Geometry check sheet. Reference: the model listing, model coordinates, mm. A direction names the side the tool comes from. Coordinates: 2 decimals unless noted, no trailing zeros. Write each loop counter-clockwise with the first axis right and the second up, starting at its lowest first coordinate (ties: lowest second). Pieces come first, ordered by that corner, then holes. Notation, with made-up numbers: (-4, 37) -> (7, 37) arc R18 ccw to (7, 44) -> close; hole circle Ø2 at (81.5, 5.25). An arc over 180 degrees is marked (long way). Answer in a Markdown table with one row per item. Add a question column.
1. Set-up check for faces 1 (the cylindrical face through (22.5, 21.5, -10)), 2 (the flat face through (0, -18, 14.5)), 3 (the cylindrical face through (22.507, -12.594, -15.281)): record each of +Z, -Z, +X, -X, +Y, -Y from which the full face is reachable in a straight line by a thin tool's end or side.
2. Cross-section at A-A on y = -4.5. Record the cut outline in (x, z).
3. Cross-section at D-D on y = 2. Record the cut outline in (x, z), and give its area (3 significant figures).
4. Mould release check, pull along Z, two halves, no side actions. Record for faces 4 (the flat face through (2, -17, 0)), 5 (the flat face through (20.6, 1, 8)), 6 (the cylindrical face through (14.23, -16.78, -1.97)): pulls with the +Z half, pulls with the -Z half, needs draft (parallel to the pull), parting line crosses it, or undercut.
5. Cross-section at C-C on y = 10. Record the cut outline in (x, z).
6. Cross-section at B-B on x = 0. Record the cut outline in (y, z), and give its area (4 significant figures).
7. Scan lines: L1, parallel to Z at x = -18, y = -17; L2, parallel to X at y = -10, z = 7; L3, parallel to X at y = -16, z = -9.5. Record each from-to range of solid material in increasing order. Write a range as from..to.
8. Depth check by flat-ended pin: P1, Ø0.8, axis at x = 22.5, y = 5, coming from the -Z side; P2, Ø2.5, axis at x = 22, z = 5.5, coming from the +Y side; P3, Ø0.5, axis at x = 22.5, z = -48, coming from the +Y side. Enter the tip coordinate at first touch or a pass-through.
```python
from build123d import *

# Parameters (mm, degrees)
F0_W         = 44
F0_H         = 42
F1_DEPTH     = 1
F3_DEPTH     = 13.5
F4_W         = 41.2
F4_H         = 40.1
F5_DEPTH     = 1
F7_DEPTH     = 25
F9_DEPTH     = 1
F11_DEPTH    = 25
F12_W        = 42
F12_H        = 15.5
F12_W_2      = 1
F12_H_2      = 9
F13_DEPTH    = 1
F14_DEPTH    = 25
F15_R        = 8
F16_T1_DEPTH = 1
F16_T3_DEPTH = 11
F16_T5_DEPTH = 11
F16_T7_DEPTH = 11
F16_T9_DEPTH = 11
F8_R         = 1.25
F17_DEPTH    = 5
F18_R        = 1


# Not quite as in the source:
# - a fillet or chamfer that OpenCascade refuses, or shapes differently, is made with other operations: its cross-section is extruded or revolved along the edge and cut away or added
# - a feature names something its author has since deleted; it is built from what else it names


with BuildPart() as f1:
    # F0 (on Top) → F1 (new body)
    with BuildSketch(Plane.XY):
        Rectangle(F0_W, F0_H)
    extrude(amount=F1_DEPTH)

    # F2 (on face) → F3 (join)
    with BuildSketch(Plane.XY.offset(1)):
        Polygon((-20.6, -19.1), (-20.6, 21), (-22, 21), (-22, -21), (22, -21), (22, 21), (20.6, 21), (20.6, -19.1), align=None)
    extrude(amount=F3_DEPTH)

    # F4 (on face) → F5 (join)
    with BuildSketch(Plane.XY.offset(14.5)):
        with Locations((0, 0.95)):
            Rectangle(F4_W, F4_H)
        Polygon((-22, 21), (-22, -21), (22, -21), (22, 21), (20.6, 21), (20.6, -19.1), (-20.6, -19.1), (-20.6, 21), align=None)
    extrude(amount=F5_DEPTH)

    # F6 (on face) → F7 (cut, symmetric)
    with BuildSketch(Plane.XY.offset(1)):
        with BuildLine():
            ThreePointArc((-20.6, 4.0000000362), (-1.81e-08, -16.6), (20.6, 4))
            ThreePointArc((20.6, 4), (18.2212690578, 13.6096490011), (11.6344316578, 21))
            Line((11.6344316578, 21), (-11.6344316578, 21))
            ThreePointArc((-11.6344316578, 21), (-18.2212690493, 13.6096490171), (-20.6, 4.0000000362))
        make_face()
        with BuildLine():
            Line((-20.6, 21), (-20.6, 4.0000000362))
            ThreePointArc((-20.6, 4.0000000362), (-18.2212690493, 13.6096490171), (-11.6344316578, 21))
            Line((-11.6344316578, 21), (-20.6, 21))
        make_face()
        with BuildLine():
            ThreePointArc((11.6344316578, 21), (18.2212690578, 13.6096490011), (20.6, 4))
            Line((20.6, 4), (20.6, 21))
            Line((20.6, 21), (11.6344316578, 21))
        make_face()
    extrude(amount=F7_DEPTH, both=True, mode=Mode.SUBTRACT)

    # F4 (on face) → F9 (join)
    with BuildSketch(Plane.XY.offset(14.5)):
        Polygon((-22, 21), (-22, -21), (22, -21), (22, 21), (20.6, 21), (20.6, -19.1), (-20.6, -19.1), (-20.6, 21), align=None)
    extrude(amount=F9_DEPTH)

    # F10 (on face) → F11 (cut)
    with BuildSketch(Plane.YZ.offset(-20.6)):
        Polygon((21, 0), (21, 15), (21, 15.5), (4, 15.5), (4, 14.5), (4, 1), (4, 0), align=None)
    extrude(amount=-F11_DEPTH, mode=Mode.SUBTRACT)

    # F12 (on face) → F13 (join)
    with BuildSketch(Plane.YZ.offset(22)):
        Polygon((21, 0), (-21, 0), (-21, -13), (-15, -13), (25, -13), (25, 0), align=None)
        with BuildLine():
            Line((23, -7.5), (23, -8.5))
            ThreePointArc((23, -8.5), (21.5, -10), (20, -8.5))
            Line((20, -8.5), (20, -7.5))
            ThreePointArc((20, -7.5), (21.5, -6), (23, -7.5))
        make_face(mode=Mode.SUBTRACT)
        Polygon((-15, -13), (-21, -13), (-21, -55), (-15, -55), (-15, -46), align=None)
        with BuildLine():
            Line((-16.45, -49.5), (-16.45, -50.5))
            ThreePointArc((-16.45, -50.5), (-18, -52.05), (-19.55, -50.5))
            Line((-19.55, -50.5), (-19.55, -49.5))
            ThreePointArc((-19.55, -49.5), (-18, -47.95), (-16.45, -49.5))
        make_face(mode=Mode.SUBTRACT)
        with Locations((0, 7.75)):
            Rectangle(F12_W, F12_H)
        with Locations((-14.5, -50.5)):
            Rectangle(F12_W_2, F12_H_2)
    extrude(amount=F13_DEPTH)

    # F12 (on face) → F14 (cut)
    with BuildSketch(Plane.YZ.offset(22)):
        with BuildLine():
            ThreePointArc((-19.55, -50.5), (-18, -52.05), (-16.45, -50.5))
            Line((-16.45, -50.5), (-16.8157280718, -50.5))
            ThreePointArc((-16.8157280718, -50.5), (-18, -51.05), (-19.1842719282, -50.5))
            Line((-19.1842719282, -50.5), (-19.55, -50.5))
        make_face()
        with BuildLine():
            Line((-16.8157280718, -50.5), (-16.45, -50.5))
            ThreePointArc((-16.45, -50.5), (-16.4708552854, -50.2465903676), (-16.5328599249, -50))
            ThreePointArc((-16.5328599249, -50), (-16.6509275769, -50.2632192327), (-16.8157280718, -50.5))
        make_face()
        with BuildLine():
            ThreePointArc((-16.5328599249, -50), (-16.4708552854, -50.2465903676), (-16.45, -50.5))
            Line((-16.45, -50.5), (-16.45, -49.5))
            ThreePointArc((-16.45, -49.5), (-16.4708552854, -49.7534096324), (-16.5328599249, -50))
        make_face()
        with BuildLine():
            ThreePointArc((-16.5328599249, -50), (-16.4708552854, -49.7534096324), (-16.45, -49.5))
            Line((-16.45, -49.5), (-16.8157280718, -49.5))
            ThreePointArc((-16.8157280718, -49.5), (-16.6509275769, -49.7367807673), (-16.5328599249, -50))
        make_face()
        with BuildLine():
            Line((-16.8157280718, -49.5), (-16.45, -49.5))
            ThreePointArc((-16.45, -49.5), (-18, -47.95), (-19.55, -49.5))
            Line((-19.55, -49.5), (-19.1842719282, -49.5))
            ThreePointArc((-19.1842719282, -49.5), (-18, -48.95), (-16.8157280718, -49.5))
        make_face()
        with BuildLine():
            Line((-19.1842719282, -49.5), (-16.8157280718, -49.5))
            ThreePointArc((-16.8157280718, -49.5), (-18, -48.95), (-19.1842719282, -49.5))
        make_face()
        with BuildLine():
            Line((-19.1842719282, -50.5), (-16.8157280718, -50.5))
            ThreePointArc((-16.8157280718, -50.5), (-16.6509275769, -50.2632192327), (-16.5328599249, -50))
            ThreePointArc((-16.5328599249, -50), (-16.6509275769, -49.7367807673), (-16.8157280718, -49.5))
            Line((-16.8157280718, -49.5), (-19.1842719282, -49.5))
            ThreePointArc((-19.1842719282, -49.5), (-19.3490724231, -49.7367807673), (-19.4671400751, -50))
            ThreePointArc((-19.4671400751, -50), (-19.3490724231, -50.2632192327), (-19.1842719282, -50.5))
        make_face()
        with BuildLine():
            ThreePointArc((-19.1842719282, -50.5), (-18, -51.05), (-16.8157280718, -50.5))
            Line((-16.8157280718, -50.5), (-19.1842719282, -50.5))
        make_face()
        with BuildLine():
            ThreePointArc((-19.4671400751, -50), (-19.5291447146, -50.2465903676), (-19.55, -50.5))
            Line((-19.55, -50.5), (-19.1842719282, -50.5))
            ThreePointArc((-19.1842719282, -50.5), (-19.3490724231, -50.2632192327), (-19.4671400751, -50))
        make_face()
        with BuildLine():
            Line((-19.55, -49.5), (-19.55, -50.5))
            ThreePointArc((-19.55, -50.5), (-19.5291447146, -50.2465903676), (-19.4671400751, -50))
            ThreePointArc((-19.4671400751, -50), (-19.5291447146, -49.7534096324), (-19.55, -49.5))
        make_face()
        with BuildLine():
            Line((-19.1842719282, -49.5), (-19.55, -49.5))
            ThreePointArc((-19.55, -49.5), (-19.5291447146, -49.7534096324), (-19.4671400751, -50))
            ThreePointArc((-19.4671400751, -50), (-19.3490724231, -49.7367807673), (-19.1842719282, -49.5))
        make_face()
        with BuildLine():
            ThreePointArc((20, -8.5), (21.5, -10), (23, -8.5))
            Line((23, -8.5), (22.6180339887, -8.5))
            ThreePointArc((22.6180339887, -8.5), (21.5, -9), (20.3819660113, -8.5))
            Line((20.3819660113, -8.5), (20, -8.5))
        make_face()
        with BuildLine():
            ThreePointArc((20.0857864376, -8), (20.0216021605, -8.2463470319), (20, -8.5))
            Line((20, -8.5), (20.3819660113, -8.5))
            ThreePointArc((20.3819660113, -8.5), (20.209430585, -8.2644805982), (20.0857864376, -8))
        make_face()
        with BuildLine():
            Line((20.3819660113, -7.5), (20, -7.5))
            ThreePointArc((20, -7.5), (20.0216021605, -7.7536529681), (20.0857864376, -8))
            ThreePointArc((20.0857864376, -8), (20.209430585, -7.7355194018), (20.3819660113, -7.5))
        make_face()
        with BuildLine():
            Line((22.6180339887, -7.5), (23, -7.5))
            ThreePointArc((23, -7.5), (21.5, -6), (20, -7.5))
            Line((20, -7.5), (20.3819660113, -7.5))
            ThreePointArc((20.3819660113, -7.5), (21.5, -7), (22.6180339887, -7.5))
        make_face()
        with BuildLine():
            Line((20.3819660113, -7.5), (22.6180339887, -7.5))
            ThreePointArc((22.6180339887, -7.5), (21.5, -7), (20.3819660113, -7.5))
        make_face()
        with BuildLine():
            Line((20.3819660113, -8.5), (22.6180339887, -8.5))
            ThreePointArc((22.6180339887, -8.5), (22.790569415, -8.2644805982), (22.9142135624, -8))
            ThreePointArc((22.9142135624, -8), (22.790569415, -7.7355194018), (22.6180339887, -7.5))
            Line((22.6180339887, -7.5), (20.3819660113, -7.5))
            ThreePointArc((20.3819660113, -7.5), (20.209430585, -7.7355194018), (20.0857864376, -8))
            ThreePointArc((20.0857864376, -8), (20.209430585, -8.2644805982), (20.3819660113, -8.5))
        make_face()
        with BuildLine():
            ThreePointArc((20.3819660113, -8.5), (21.5, -9), (22.6180339887, -8.5))
            Line((22.6180339887, -8.5), (20.3819660113, -8.5))
        make_face()
        with BuildLine():
            ThreePointArc((22.9142135624, -8), (22.9783978395, -8.2463470319), (23, -8.5))
            Line((23, -8.5), (23, -7.5))
            ThreePointArc((23, -7.5), (22.9783978395, -7.7536529681), (22.9142135624, -8))
        make_face()
        with BuildLine():
            ThreePointArc((22.9142135624, -8), (22.9783978395, -7.7536529681), (23, -7.5))
            Line((23, -7.5), (22.6180339887, -7.5))
            ThreePointArc((22.6180339887, -7.5), (22.790569415, -7.7355194018), (22.9142135624, -8))
        make_face()
        with BuildLine():
            Line((22.6180339887, -8.5), (23, -8.5))
            ThreePointArc((23, -8.5), (22.9783978395, -8.2463470319), (22.9142135624, -8))
            ThreePointArc((22.9142135624, -8), (22.790569415, -8.2644805982), (22.6180339887, -8.5))
        make_face()
        with BuildLine():
            Line((20, -7.5), (20, -8.5))
            ThreePointArc((20, -8.5), (20.0216021605, -8.2463470319), (20.0857864376, -8))
            ThreePointArc((20.0857864376, -8), (20.0216021605, -7.7536529681), (20, -7.5))
        make_face()
    extrude(amount=-F14_DEPTH, mode=Mode.SUBTRACT)

    # F15
    f15_edges = [f1.edges().sort_by_distance(p)[0] for p in [
        (22.5, -15, -13),
    ]]
    fillet(f15_edges, radius=F15_R)

    # F16: fillet of radius 2 on 5 edges, made by hand

    # F16_s2 → F16_t1 (join)
    with BuildSketch(Plane.YZ.offset(22)):
        with BuildLine():
            ThreePointArc((-15, -44.2679491924), (-14.7320508076, -45.2679491924), (-14, -46))
            Line((-14, -46), (-15, -46))
            Line((-15, -46), (-15, -44.2679491924))
        make_face()
    extrude(amount=F16_T1_DEPTH)

    # F16_s4 → F16_t3 (cut)
    with BuildSketch(Plane.YZ.offset(17)):
        with BuildLine():
            ThreePointArc((23, -13), (24.4142135624, -12.4142135624), (25, -11))
            Line((25, -11), (25, -13))
            Line((25, -13), (23, -13))
        make_face()
    extrude(amount=F16_T3_DEPTH, mode=Mode.SUBTRACT)

    # F16_s6 → F16_t5 (cut)
    with BuildSketch(Plane.YZ.offset(17)):
        with BuildLine():
            ThreePointArc((23, 0), (24.4142135624, -0.5857864376), (25, -2))
            Line((25, -2), (25, 0))
            Line((25, 0), (23, 0))
        make_face()
    extrude(amount=F16_T5_DEPTH, mode=Mode.SUBTRACT)

    # F16_s8 → F16_t7 (cut)
    with BuildSketch(Plane.YZ.offset(17)):
        with BuildLine():
            ThreePointArc((-14, -53), (-14.5857864376, -54.4142135624), (-16, -55))
            Line((-16, -55), (-14, -55))
            Line((-14, -55), (-14, -53))
        make_face()
    extrude(amount=F16_T7_DEPTH, mode=Mode.SUBTRACT)

    # F16_s10 → F16_t9 (cut)
    with BuildSketch(Plane.YZ.offset(17)):
        with BuildLine():
            ThreePointArc((-19, -55), (-20.4142135624, -54.4142135624), (-21, -53))
            Line((-21, -53), (-21, -55))
            Line((-21, -55), (-19, -55))
        make_face()
    extrude(amount=F16_T9_DEPTH, mode=Mode.SUBTRACT)

    # F8 (on face) → F17 (join)
    with BuildSketch(Plane(origin=(0, 0, 0), x_dir=(1, 0, 0), z_dir=(0, 0, -1))):
        with Locations((-17, 18)):
            Circle(F8_R)
        with Locations((14.5, 18)):
            Circle(F8_R)
    extrude(amount=F17_DEPTH)

    # F18
    f18_edges = [f1.edges().sort_by_distance(p)[0] for p in [
        (-18.25, -18, -5),
        (13.25, -18, -5),
        (22.5, -14, -46),
    ]]
    fillet(f18_edges, radius=F18_R)


solid = f1.part
```
Results found:
| question | item | result |
|---|---|---|
| 1 | face 1 | +X, -X |
| 1 | face 2 | +Y |
| 1 | face 3 | +X, -X, +Y |
| 2 | outline | (-22, 0) -> (-18.76, 0) -> (-18.76, 1) -> (-20.6, 1) -> (-20.6, 14.5) -> (-18.76, 14.5) -> (-18.76, 15.5) -> (-22, 15.5) -> close; (18.76, 0) -> (22, 0) -> (22, -13) -> (23, -13) -> (23, 15.5) -> (18.76, 15.5) -> (18.76, 14.5) -> (20.6, 14.5) -> (20.6, 1) -> (18.76, 1) -> close |
| 3 | outline | (-22, 0) -> (-20.5, 0) -> (-20.5, 1) -> (-20.6, 1) -> (-20.6, 14.5) -> (-20.5, 14.5) -> (-20.5, 15.5) -> (-22, 15.5) -> close; (20.5, 0) -> (22, 0) -> (22, -13) -> (23, -13) -> (23, 15.5) -> (20.5, 15.5) -> (20.5, 14.5) -> (20.6, 14.5) -> (20.6, 1) -> (20.5, 1) -> close |
| 3 | area | 72.3 mm^2 |
| 4 | face 4 | pulls with the -Z half |
| 4 | face 5 | undercut |
| 4 | face 6 | needs draft |
| 5 | outline | (20.6, 0) -> (22, 0) -> (22, -13) -> (23, -13) -> (23, 15.5) -> (20.6, 15.5) -> close |
| 6 | outline | (-21, 0) -> (-16.6, 0) -> (-16.6, 1) -> (-19.1, 1) -> (-19.1, 14.5) -> (-16.6, 14.5) -> (-16.6, 15.5) -> (-21, 15.5) -> close |
| 6 | area | 34.45 mm^2 |
| 7 | L1 | z = 0..1, 14.5..15.5 |
| 7 | L2 | x = -22..-20.6, 20.6..23 |
| 7 | L3 | x = 22..23 |
| 8 | P1 | stops at z = -13 |
| 8 | P2 | stops at y = 21 |
| 8 | P3 | stops at y = -14 |
